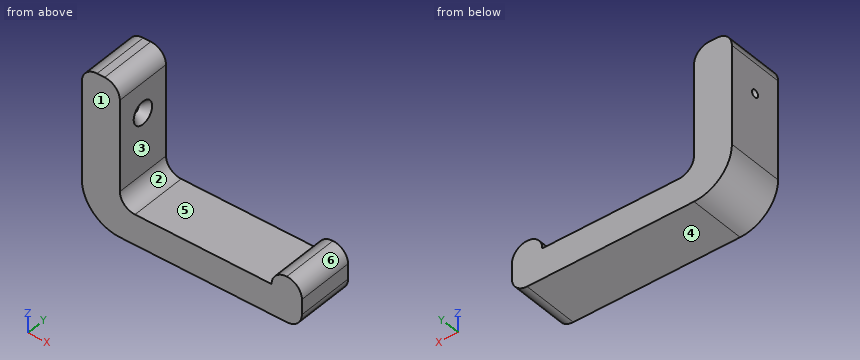
from build123d import *

# Parameters (mm, degrees)
F0_W           = 40
F0_H           = 8
F1_DEPTH       = 15
F2_R           = 3.99999
F3_R           = 10
F5_D           = 2
F5_CSINK_D     = 6
F5_CSINK_ANGLE = 90


# Not quite as in the source:
# - a fillet or chamfer is up to 0.001 mm smaller than in the source, because OpenCascade refuses the exact size


with BuildPart() as f1:
    # F0 (on Front) → F1 (new body)
    with BuildSketch(Plane.XZ):
        Polygon((-20, -4), (-20, 4), (-20, 36), (-30, 36), (-30, -4), align=None)
        Rectangle(F0_W, F0_H)
        Polygon((20, 8), (20, 4), (20, -4), (28, -4), (28, 8), align=None)
    extrude(amount=F1_DEPTH)

    # F2 (radius 4 in the source; OpenCascade refuses exactly that, so slightly less here)
    f2_edges = [f1.edges().sort_by_distance(p)[0] for p in [
        (-20, -7.5, 4),
        (20, -7.5, 8),
        (28, -7.5, 8),
        (28, -7.5, -4),
        (-20, -7.5, 36),
        (-30, -7.5, 36),
    ]]
    fillet(f2_edges, radius=F2_R)

    # F3
    f3_edges = [f1.edges().sort_by_distance(p)[0] for p in [
        (-30, -7.5, -4),
    ]]
    fillet(f3_edges, radius=F3_R)

    # F5 (through all)
    with Locations(Plane.YZ.offset(-20)):
        with Locations((-7.5, 24)):
            CounterSinkHole(F5_D / 2, F5_CSINK_D / 2, counter_sink_angle=F5_CSINK_ANGLE)


solid = f1.part
Check sheet for the modelled part. Datum: model origin and axes. Units: mm. Face numbers are marked on the shaded views. A direction names the side the tool comes from. Round coordinates to 2 decimals unless told otherwise and drop trailing zeros. Order: outer loops, then holes, each group sorted by start corner. A loop starts at its lowest first (then second) coordinate and runs counter-clockwise, first axis right, second up.
(1) Cross-section at D-D, the plane z = 19. Enter the section's corners in (x, y).
(2) Cross-section at C-C, the plane x = -21. Enter the section's corners in (y, z).
(3) Go/stop test with flat-tipped pins: P1, Ø8, axis at x = -13, z = 24, coming from the +Y side; P2, Ø4.5, axis at x = -0.5, y = -9.5, coming from the +Z side; P3, Ø7.5, axis at y = -4, z = 19, coming from the +X side. Record where each tip stops, or that it passes through.
(4) Access from +Z, -Z, +X, -X, +Y, -Y to the whole of each face (thin tool, end or side, straight path). Record for the marked faces 1, 2 and 3.
(5) Cross-section at B-B, the plane z = 24. Enter the section's corners in (x, y).
(6) Draft check along X on the marked faces 4, 5 and 6. Enter one of: pulls with the +X half, pulls with the -X half, needs draft (parallel to the pull), parting line crosses it, or undercut.
(7) Scan lines: probe 1 along Y at (x, z) = (-28, 24); probe 2 along X at (y, z) = (-5, 18); probe 3 along Z at (x, y) = (0.5, -5.75). Record each from-to range of solid material in increasing order.
Check sheet entries:
1. outline: (-30, -15) - (-20, -15) - (-20, 0) - (-30, 0) - close
2. outline: (-15, -3.95) - (0, -3.95) - (0, 34.65) - (-15, 34.65) - close; hole circle Ø4 at (-7.5, 24)
3. P1: passes through
3. P2: stops at z = 4
3. P3: stops at x = -20
4. face 1: +Z, -Z, +X, -X, -Y
4. face 2: +Z, +Y, -Y
4. face 3: +Z, +X, +Y, -Y
5. outline: (-30, -15) - (-20, -15) - (-20, -10.5) - (-22, -8.5) - (-30, -8.5) - close; (-30, -6.5) - (-22, -6.5) - (-20, -4.5) - (-20, 0) - (-30, 0) - close
6. face 4: needs draft
6. face 5: undercut
6. face 6: pulls with the +X half
7. probe 1: y = -15 to -8.5, -6.5 to 0
7. probe 2: x = -30 to -20
7. probe 3: z = -4 to 4
